Autodesk Inventor part; units mm, degrees
ref_plane "Work Plane1" through (16.3751, 0, 0) normal (0, 0, 1) x (-1, 0, 0)
ref_plane "YZ Plane" through (0, 0, 0) normal (1, 0, 0) x (0, 1, 0)
ref_plane "XZ Plane" through (0, 0, 0) normal (0, 1, 0) x (-1, 0, 0)
sketch "Sketch1" plane through (0, 0, 0) normal (1, 0, 0) x (0, 1, 0)
  line L0 (-5.7735, 0) -> (-2.8868, 5)
  line L1 (-2.8868, 5) -> (2.8868, 5)
  line L2 (2.8868, 5) -> (5.7735, 0)
  line L3 (5.7735, 0) -> (2.8868, -5)
  line L4 (2.8868, -5) -> (-2.8868, -5)
  line L5 (-2.8868, -5) -> (-5.7735, 0)
  point P0 (0, 0)
  point P1 (0, 0)
  dimension "d0" = 11.547
extrude "Body" add sketch "Sketch1" along normal blind 5.9
sketch "Sketch2" plane through (0, 0, 0) normal (-1, 0, 0) x (0, 0, 1)
  line L0 (0, -8.0829) -> (0, 8.0829)
  line L1 (-7, 0) -> (7, 0)
  point P0 (0, 0)
hole "Thread" at (0, 0, 0) direction (1, 0, 0) diameter 4.917 end through all
chamfer "Chamfer1" distance 0.5413 angle 30 1 edges at (0, 0, -2.4585) measured on face at (0, -3.5612, -2.1322)
chamfer "Chamfer2" distance 0.5413 angle 30 1 edges at (5.9, 0, -2.4585) measured on face at (5.9, -3.5612, -2.1322)
sketch "Sketch3" plane through (0, 0, 0) normal (0, 0, 1) x (1, 0, 0)
  line L0 (0, 2.8868) -> (0, 5.7735)
  line L1 (0, 5.7735) -> (5.9, 5.7735)
  line L2 (5.9, 2.8868) -> (5.9, 5.7735)
  line L3 (-1.18, 0) -> (7.08, 0)
  line L4 (0.4466, 5.7735) -> (0, 5)
  line L5 (5.9, 4.25) -> (4.8156, 4.25)
  line L6 (4.8156, 4.25) -> (3, 5.7735)
  dimension "d3" = 30
  dimension "d5" = 10
  dimension "d6" = 8.5
  dimension "d8" = 50
  dimension "d9" = 3
revolve "Chamfer3" cut sketch "Sketch3" angle 360 about axis through (-10, 0, 0) along (1, 0, 0)
ref_plane "Work Plane1" through (16.3751, 0, 0) normal (0, 0, 1) x (-1, 0, 0)
equation "\"d0\" = 1.1547 * SW"
equation "\"d1\" = KOH"
equation "\"d3\" = ANG1"
equation "\"d5\" = SW0"
equation "\"d6\" = SW1"
equation "\"d8\" = ANG2"
equation "\"d9\" = KOH1"
equation "\"d10\" = -0.5 * GD1 + 0.5 * NND"
equation "\"d39\" = -0.5 * GD1 + 0.5 * NND"
equation "\"d12\" = -0.5 * GD1 + 0.5 * NND"
equation "\"d40\" = -0.5 * GD1 + 0.5 * NND"
equation "\"ANG1\" = 30deg"
equation "\"ANG2\" = 50deg"
equation "\"NND\" = 6"
equation "\"KOH\" = 5.9"
equation "\"SW0\" = SW"
equation "\"SW1\" = 0.85 * SW"
equation "\"KOH1\" = 3"
equation "\"GUL\" = 0.541266 * PTC"
equation "\"THREADDIA\" = 6"
equation "\"TOA\" = 30deg"
equation "\"PTC\" = 1"
equation "\"E0\" = 1.155 * SW"
equation "\"GAL\" = 0.541266 * PTC"
properties part number "ANSI B18.16.3M - Property Class 5 and 10 - Metric M6 x 1 Metal Type" material "Steel, Mild"
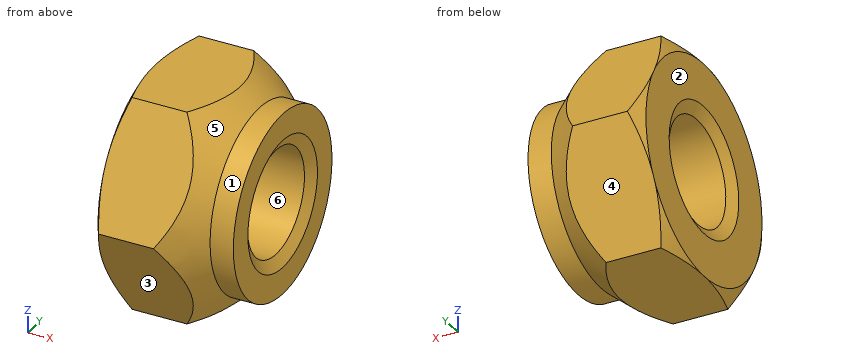
Could you check a few things on this model? Use its own coordinates, in mm. Face numbers are marked on the shaded views. A direction names the side the tool comes from. Coordinates: 2 decimals unless noted, no trailing zeros. Write each loop counter-clockwise with the first axis right and the second up, starting at its lowest first coordinate (ties: lowest second). Pieces come first, ordered by that corner, then holes. Notation, with made-up numbers: (-6, 61) -> (32, 61) arc R20 ccw to (32, 65) -> close; hole circle Ø8 at (67, -32). An arc over 180 degrees is marked (long way). One line per question, with ' | ' between items. Start each with the question number.
1. If we section it at B-B (x = 4.4): Please give me the cut outline in (y, z).
2. For the marked faces 1 and 2, which set-ups out of +Z, -Z, +X, -X, +Y, -Y let a thin tool reach every point of the face, with its end or its side?
3. Thinking about a two-plate mould opening in Y: for the marked faces 3, 4, 5 and 6, which applies, pulls with the +Y half, pulls with the -Y half, needs draft (parallel to the pull), parting line crosses it, or undercut?
4. Please list where these lines run through material, in increasing order: line 1 along Z through (x, y) = (3.65, 0); line 2 along Z through (x, y) = (4, 0); line 3 along Y through (x, z) = (1.75, -2.25).
5. If we section it at A-A (x = 1.15): Please give me the cut outline in (y, z), and give its area (3 significant figures).
6. Will this pin go through, and if not, where does the flat tip stop? P1, Ø1, axis at y = 3.5, z = -3.5, coming from the +X side.
Return value:
1) outline: circle Ø9.2 at (0, 0); hole circle Ø4.92 at (0, 0)
2) face 1: +X | face 2: +Z, -Z, -X, +Y, -Y
3) face 3: pulls with the -Y half | face 4: pulls with the +Y half | face 5: parting line crosses it | face 6: undercut
4) line 1: z = -5 to -2.46, 2.46 to 5 | line 2: z = -4.93 to -2.46, 2.46 to 4.93 | line 3: y = -4.47 to -0.99, 0.99 to 4.47
5) outline: (-5.77, 0) -> (-2.89, -5) -> (2.89, -5) -> (5.77, 0) -> (2.89, 5) -> (-2.89, 5) -> close; hole circle Ø4.92 at (0, 0) | area: 67.6 mm²
6) P1: stops at x = 4.58
